Model file for the job. Use its own axes, mm. A direction names the side the tool comes from. Give positions to 0.01 mm unless a question says otherwise; leave off trailing zeros. Loops run counter-clockwise (first coordinate to the right, second up) from the corner with the lowest first, then second, coordinate; pieces in that order, holes last. Notation, with made-up numbers: (42.5, 73.25) - (91.5, 73.25) arc R17 ccw to (91.5, 105.25) - close; hole circle Ø9 at (71.25, 59). An arc over 180 degrees is marked (long way). Answer as CSV lines item,"result". Start each with the question number.
Item 1: Drill centre lines: L1, parallel to Y at x = -12.7, z = 9.5; L2, parallel to Z at x = -5, y = 0.25; L3, parallel to X at y = 3.5, z = 30. Where is each one in solid material? Low to high. Write a range as from..to.
Item 2: Saw through at D-D on x = -24. Give the cut face in (y, z).
Item 3: Tool access for faces 1 (the cylindrical face through (-12.97, 4.91, 97.54)), 2 (the flat face through (-13, 10, 50.837)), 3 (the flat face through (-13, 13.05, 80)), 4 (the flat face through (-13, 0, 17.78)), 5 (the cylindrical face through (-3.055, 0.528, 106.323)): list every direction of +Z, -Z, +X, -X, +Y, -Y with a clear straight run to the whole face (end or side of a thin tool).
Item 4: Saw through at B-B on x = -6.35. Give the cut face in (y, z).
Item 5: Saw through at A-A on y = 10. State how many separate pieces and enclosed holes the cut face has, plus the area to 3 significant figures.
Item 6: Pin check, flat tips, straight feed: pin 1 (3 mm diameter, centred on x = -8.5, y = 10, fed in from -Z); pin 2 (1.9 mm diameter, centred on x = -18, y = 11, fed in from +Z); pin 3 (7.5 mm diameter, centred on x = -18, z = 18.5, fed in from +Y). Stop position of each tip, or through.
Item 7: Pull direction Z, two halves, no side cores. Call faces 6 (the cylindrical face through (-5.396, 0.528, 89.913)), 7 (the flat face through (-25.4, 0, 49)), 8 (the flat face through (-13, 3, 0)): pulls with the +Z half, pulls with the -Z half, needs draft (parallel to the pull), parting line crosses it, or undercut.
from build123d import *

# Parameters (mm, degrees)
SKETCH1_W           = 25.4
SKETCH1_H           = 25.4
BOSS_EXTRUDE1_DEPTH = 109.22
SKETCH2_R           = 2.54
CUT_EXTRUDE1_DEPTH  = 17.78
SKETCH3_R           = 4.7625
CUT_EXTRUDE2_DEPTH  = 115.975338225
SKETCH7_W           = 25.4
SKETCH7_H           = 9.525
CUT_EXTRUDE5_DEPTH  = 6.35
SKETCH9_R           = 3.175
CUT_EXTRUDE7_DEPTH  = 115.975338225
SKETCH10_R          = 3.81
CUT_EXTRUDE8_DEPTH  = 16.51
FILLET1_R           = 10.16
FILLET2_R           = 10.16


with BuildPart() as part:
    # Sketch1 → Boss-Extrude1 (new body)
    with BuildSketch(Plane.XY):
        with Locations((-12.7, 0.350344828)):
            Rectangle(SKETCH1_W, SKETCH1_H)
    extrude(amount=BOSS_EXTRUDE1_DEPTH)

    # Sketch2 → Cut-Extrude1 (cut)
    with BuildSketch(Plane(origin=(0, 0, 0), x_dir=(-1, 0, 0), z_dir=(0, 0, -1))):
        with Locations((12.7, 0)):
            Circle(SKETCH2_R)
    extrude(amount=-CUT_EXTRUDE1_DEPTH, mode=Mode.SUBTRACT)

    # Sketch3 → Cut-Extrude2 (cut, through all)
    with BuildSketch(Plane(origin=(0, 13.050344828, 0), x_dir=(1, 0, 0), z_dir=(0, 1, 0))):
        with Locations(Location((-12.7, -32.385, 0), (0, 0, 270))):
            Circle(SKETCH3_R)
    extrude(amount=-CUT_EXTRUDE2_DEPTH, mode=Mode.SUBTRACT)

    # Sketch7 → Cut-Extrude5 (cut)
    with BuildSketch(Plane(origin=(0, 13.050344828, 0), x_dir=(1, 0, 0), z_dir=(0, 1, 0))):
        with Locations((-12.7, -18.695040466)):
            Rectangle(SKETCH7_W, SKETCH7_H)
        with Locations((-12.7, -46.074959534)):
            Rectangle(SKETCH7_W, SKETCH7_H)
    extrude(amount=-CUT_EXTRUDE5_DEPTH, mode=Mode.SUBTRACT)

    # Sketch9 → Cut-Extrude7 (cut, through all)
    with BuildSketch(Plane(origin=(0, 13.050344828, 0), x_dir=(1, 0, 0), z_dir=(0, 1, 0))):
        with Locations(Location((-19.05, -86.884321607, 0), (0, 0, 270))):
            Circle(SKETCH9_R)
        with Locations(Location((-6.35, -86.884321607, 0), (0, 0, 270))):
            Circle(SKETCH9_R)
    extrude(amount=-CUT_EXTRUDE7_DEPTH, mode=Mode.SUBTRACT)

    # Sketch10 → Cut-Extrude8 (cut)
    with BuildSketch(Plane(origin=(0, 13.050344828, 0), x_dir=(1, 0, 0), z_dir=(0, 1, 0))):
        with Locations(Location((-13.13594772, -101.346, 0), (0, 0, 270))):
            Circle(SKETCH10_R)
    extrude(amount=-CUT_EXTRUDE8_DEPTH, mode=Mode.SUBTRACT)

    # Fillet1
    fillet1_edges = [part.edges().sort_by_distance(p)[0] for p in [
        (0, 0.350344828, 109.22),
    ]]
    fillet(fillet1_edges, radius=FILLET1_R)

    # Fillet2
    fillet2_edges = [part.edges().sort_by_distance(p)[0] for p in [
        (-25.4, 0.350344828, 109.22),
    ]]
    fillet(fillet2_edges, radius=FILLET2_R)


solid = part.part
Responses:
1,L1,"-12.35..-2.54, 2.54..13.05"
1,L2,"0..84.01, 89.76..107.81"
1,L3,"-25.4..-16.82, -8.58..0"
2,outline,"(-12.35, 0) - (13.05, 0) - (13.05, 13.93) - (6.7, 13.93) - (6.7, 23.46) - (13.05, 23.46) - (13.05, 41.31) - (6.7, 41.31) - (6.7, 50.84) - (13.05, 50.84) - (13.05, 104.21) - (-12.35, 104.21) - close"
3,face 1,"+Y"
3,face 2,"+X, -X, +Y"
3,face 3,"+Z, -Z, +X, -X, +Y"
3,face 4,"-Z"
3,face 5,"+Z, +X, +Y, -Y"
4,outline,"(-12.35, 0) - (13.05, 0) - (13.05, 13.93) - (6.7, 13.93) - (6.7, 23.46) - (13.05, 23.46) - (13.05, 41.31) - (6.7, 41.31) - (6.7, 50.84) - (13.05, 50.84) - (13.05, 83.71) - (-12.35, 83.71) - close; (-12.35, 90.06) - (13.05, 90.06) - (13.05, 108.48) - (-12.35, 108.48) - close"
5,separate pieces,"3"
5,enclosed holes,"4"
5,area,"2,070 mm2"
6,pin 1,"z = 0"
6,pin 2,"z = 109.06"
6,pin 3,"y = 6.7"
7,face 6,"undercut"
7,face 7,"needs draft"
7,face 8,"pulls with the -Z half"
